Design review of the part built by this model. Coordinates are the model's own, in mm. A direction names the side the tool comes from. Round coordinates to 2 decimals unless told otherwise and drop trailing zeros. Loops run counter-clockwise (first coordinate to the right, second up) from the corner with the lowest first, then second, coordinate; pieces in that order, holes last. Notation, with made-up numbers: (-6, -29) - (41, -29) arc R18 ccw to (41, -12) - close; hole circle Ø6 at (13, 64). An arc over 180 degrees is marked (long way). Return JSON: item names as keys, results as strings. Group by question number.
(1) For faces 1 (the flat face through (-55.9, -3, 3)), 2 (the flat face through (-66.4, 0, 0)), list the 3-axis set-ups (+Z, -Z, +X, -X, +Y, -Y) from which the entire face can be reached by the end or side of a thin tool; tool diameter is ignored.
(2) We need section A-A, the plane y = 0. Write out the cut boundary in (x, z), and give its area (3 significant figures).
(3) Wall thickness on L1, parallel to X at y = -7, z = 3.25; L2, parallel to Z at x = -54, y = 10.25; L3, parallel to Y at x = -55, z = 10.5: over which ranges is each line inside the solid? List them lowest first. Write a range as [from, to].
(4) Clearance check with flat-ended pins moving along their axes: pin 1 (4 mm diameter, centred on x = -58, z = -7.5, fed in from -Y); pin 2 (8 mm diameter, centred on x = -38.5, z = 8.5, fed in from +Y); pin 3 (3 mm diameter, centred on x = -22, y = -7.5, fed in from -Z); pin 4 (4 mm diameter, centred on y = -8, z = 5.5, fed in from -X). State where each tip first meets the part, or that it passes through.
(5) We need section D-D, the plane z = -6.75. Write out the cut boundary in (x, y), and give its area (3 significant figures).
(6) We need section C-C, the plane x = -44. Write out the cut boundary in (y, z).
from build123d import *

# Parameters (mm, degrees)
SKICA2_W   = 8.5
SKICA2_H   = 2
SKICA2_W_2 = 55.9
SKICA2_H_2 = 12.2


with BuildPart() as part:
    # Skica2 → Rotovat1 (revolve)
    with BuildSketch(Plane.XY):
        with Locations((-62.15, 1)):
            Rectangle(SKICA2_W, SKICA2_H)
        Polygon((-57.9, 0), (-55.9, 0), (-55.9, 3.5), (-57.9, 3.5), (-57.9, 2), align=None)
        with Locations((-27.95, 6.1)):
            Rectangle(SKICA2_W_2, SKICA2_H_2)
    revolve(axis=Axis((0, 0, 0), (-1, 0, 0)))


solid = part.part
Solutions:
{
 "1": {"face 1": "-X", "face 2": "+Z, -Z, -X, +Y, -Y"},
 "2": {"outline": "(-66.4, -2) - (-57.9, -2) - (-57.9, -3.5) - (-55.9, -3.5) - (-55.9, -12.2) - (0, -12.2) - (0, 12.2) - (-55.9, 12.2) - (-55.9, 3.5) - (-57.9, 3.5) - (-57.9, 2) - (-66.4, 2) - close", "area": "1,410 mm^2"},
 "3": {"L1": "[-55.9, 0]", "L2": "[-6.62, 6.62]", "L3": "[-6.21, 6.21]"},
 "4": {"pin 1": "through", "pin 2": "y = 11.34", "pin 3": "z = -10.62", "pin 4": "x = -55.9"},
 "5": {"outline": "(-55.9, -10.16) - (0, -10.16) - (0, 10.16) - (-55.9, 10.16) - close", "area": "1,140 mm^2"},
 "6": {"outline": "circle Ø24.4 at (0, 0)"}
}
